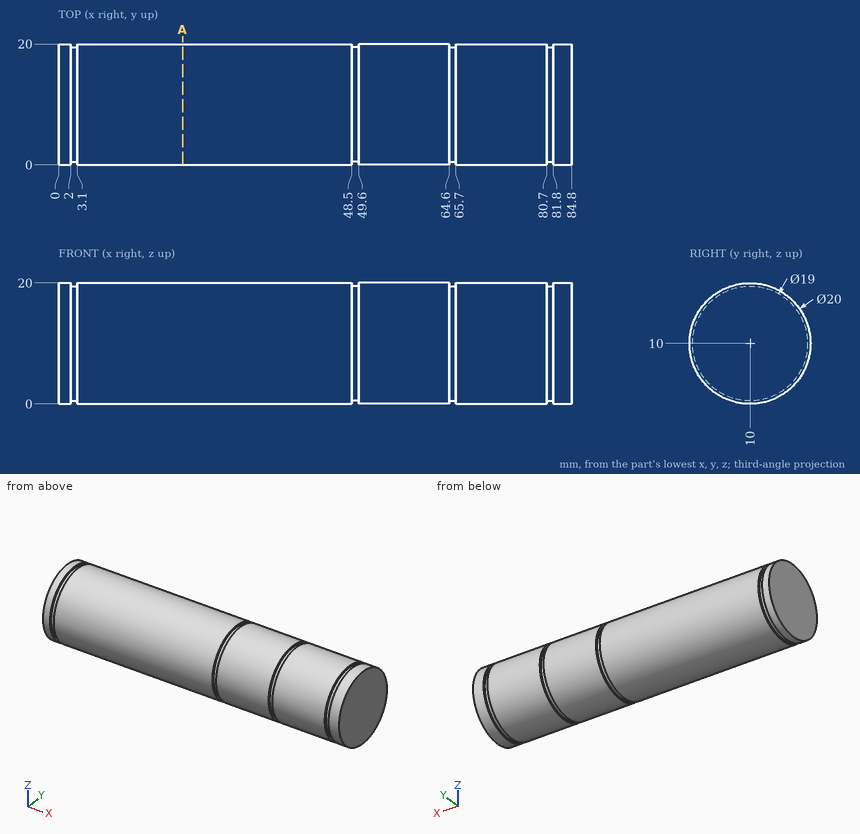
Print and shaded views of the part. All mm, measured from the part's lowest x, y and z. Coordinates: 2 decimals unless noted, no trailing zeros. Order: outer loops, then holes, each group sorted by start corner. A loop starts at its lowest first (then second) coordinate and runs counter-clockwise, first axis right, second up. Notation, with made-up numbers: M 50.5,18.5 L 73.5,18.5 A32 ccw 73.5,46.5 Z; hole C 30,74.25 d1. An arc over 180 degrees is marked long. Write each question's results on one line, items separated by ' | '. Start each with the question number.
Q1. Cut at A-A (x = 20.5). List the corners of the cut face in (y, z), then the cut area to 3 significant figures.
Q2. Drill centre lines: probe 1 along Z at (x, y) = (76.5, 9); probe 2 along Y at (x, z) = (11, 12.5); probe 3 along Y at (x, z) = (61, 5.75). Where is each one in solid material? Low to high. Write a range as from..to.
Q3. Flat gauge pins, fed straight in: P1, Ø3, axis at x = 46, z = 17, coming from the +Y side; P2, Ø4, axis at x = 74.5, z = 14.5, coming from the +Y side; P3, Ø4, axis at x = 21, z = 5, coming from the +Y side. Where does each tip first touch, or does it go through?
Found:
1) outline: C 10,10 d20 | area: 314 mm²
2) probe 1: 0.05..19.95 | probe 2: 0.32..19.68 | probe 3: 0.95..19.05
3) P1: y = 18.35 | P2: y = 19.68 | P3: y = 19.54
